from build123d import *

# Parameters (mm, degrees)
SKETCH_1_W          = 220
SKETCH_1_H          = 70
EXTRUDE_1_DEPTH     = 30
SKETCH_2_W          = 190
SKETCH_2_H          = 50
CUT_EXTRUDE_1_DEPTH = 30
SKETCH_3_W          = 20
SKETCH_3_H          = 40
CUT_EXTRUDE_2_DEPTH = 30
CUT_EXTRUDE_3_DEPTH = 30
SKETCH_5_W          = 20
SKETCH_5_H          = 60
CUT_EXTRUDE_4_DEPTH = 30
SKETCH_6_W          = 20
SKETCH_6_H          = 20
CUT_EXTRUDE_5_DEPTH = 30
SKETCH_7_W          = 20
SKETCH_7_H          = 20
CUT_EXTRUDE_6_DEPTH = 10
FILLET_1_R          = 20
EXTRUDE_2_DEPTH     = 22
EXTRUDE_3_DEPTH     = 10
EXTRUDE_START       = 10
EXTRUDE_4_DEPTH     = 10
CUT_EXTRUDE_7_DEPTH = 10
CUT_EXTRUDE_8_DEPTH = 299


with BuildPart() as part:
    # 草图1 → 凸台-拉伸1 (new body)
    with BuildSketch(Plane.XY):
        Rectangle(SKETCH_1_W, SKETCH_1_H)
    extrude(amount=EXTRUDE_1_DEPTH)

    # 草图2 → 切除-拉伸1 (cut)
    with BuildSketch(Plane.XY.offset(30)):
        with Locations((15, -10)):
            Rectangle(SKETCH_2_W, SKETCH_2_H)
    extrude(amount=-CUT_EXTRUDE_1_DEPTH, mode=Mode.SUBTRACT)

    # 草图3 → 切除-拉伸2 (cut)
    with BuildSketch(Plane(origin=(-80, 0, 0), x_dir=(0, 0, -1), z_dir=(1, 0, 0))):
        with Locations((-15, -35)):
            Rectangle(SKETCH_3_W, SKETCH_3_H)
    extrude(amount=-CUT_EXTRUDE_2_DEPTH, mode=Mode.SUBTRACT)

    # 草图4 → 切除-拉伸3 (cut)
    with BuildSketch(Plane.XY.offset(30)):
        Polygon((110, 35), (90, 15), (110, 15), align=None)
    extrude(amount=-CUT_EXTRUDE_3_DEPTH, mode=Mode.SUBTRACT)

    # 草图5 → 切除-拉伸4 (cut)
    with BuildSketch(Plane(origin=(37.5, -37.5, 0), x_dir=(0, 0, -1), z_dir=(0.7071067811865536, -0.7071067811865415, 0))):
        with Locations((-15, 102.530483272)):
            Rectangle(SKETCH_5_W, SKETCH_5_H)
    extrude(amount=-CUT_EXTRUDE_4_DEPTH, mode=Mode.SUBTRACT)

    # 草图6 → 切除-拉伸5 (cut)
    with BuildSketch(Plane(origin=(0, 35, 0), x_dir=(1, 0, 0), z_dir=(0, 1, 0))):
        with Locations((77.573593129, -15)):
            Rectangle(SKETCH_6_W, SKETCH_6_H)
    extrude(amount=-CUT_EXTRUDE_5_DEPTH, mode=Mode.SUBTRACT)

    # 草图7 → 切除-拉伸6 (cut)
    with BuildSketch(Plane(origin=(67.573593129, 0, 0), x_dir=(0, 0, -1), z_dir=(1, 0, 0))):
        with Locations((-15, 25)):
            Rectangle(SKETCH_7_W, SKETCH_7_H)
    extrude(amount=-CUT_EXTRUDE_6_DEPTH, mode=Mode.SUBTRACT)

    # 圆角1
    fillet_1_edges = [part.edges().sort_by_distance(p)[0] for p in [
        (-80, 15, 15),
    ]]
    fillet(fillet_1_edges, radius=FILLET_1_R)

    # 草图8 → 凸台-拉伸2 (add)
    with BuildSketch(Plane(origin=(0, 0, 25), x_dir=(-1, 0, 0), z_dir=(0, 0, -1))):
        Polygon((-57.573593129, 15), (-77.573593129, 35), (-57.573593129, 35), align=None)
    extrude(amount=EXTRUDE_2_DEPTH)

    # 草图9 → 凸台-拉伸3 (add)
    with BuildSketch(Plane.XY.offset(30)):
        with BuildLine():
            Line((90, 15), (110, 35))
            Line((110, 35), (-110, 35))
            Line((-110, 35), (-110, -35))
            Line((-110, -35), (-80, -35))
            Line((-80, -35), (-80, -5))
            ThreePointArc((-80, -5), (-74.142135624, 9.142135624), (-60, 15))
            Line((-60, 15), (90, 15))
        make_face()
    extrude(amount=EXTRUDE_3_DEPTH)

    # 草图10 → 凸台-拉伸4 (add)
    with BuildSketch(Plane(origin=(0, 0, 0), x_dir=(-1, 0, 0), z_dir=(0, 0, -1)).offset(EXTRUDE_START)):
        with BuildLine():
            Line((110, 35), (-110, 35))
            Line((-110, 35), (-90, 15))
            Line((-90, 15), (60, 15))
            ThreePointArc((60, 15), (74.142135624, 9.142135624), (80, -5))
            Line((80, -5), (80, -35))
            Line((80, -35), (110, -35))
            Line((110, -35), (110, 35))
        make_face()
    extrude(amount=-EXTRUDE_4_DEPTH)

    # 草图11 → 切除-拉伸7 (cut)
    with BuildSketch(Plane.XZ.offset(-15)):
        with BuildLine():
            Line((-47.5, 25), (37.5, 25))
            ThreePointArc((37.5, 25), (47.5, 15), (37.5, 5))
            Line((37.5, 5), (-47.5, 5))
            ThreePointArc((-47.5, 5), (-57.5, 15), (-47.5, 25))
        make_face()
    extrude(amount=-CUT_EXTRUDE_7_DEPTH, mode=Mode.SUBTRACT)

    # 草图12 → 切除-拉伸8 (cut)
    with BuildSketch(Plane.ZY.offset(110)):
        Polygon((-10, 31), (-5, 26), (-10, 21), align=None)
        Polygon((40, 31), (35, 26), (40, 21), align=None)
    extrude(amount=-CUT_EXTRUDE_8_DEPTH, mode=Mode.SUBTRACT)


solid = part.part
Geometry check sheet. Reference: the model listing, model coordinates, mm. A direction names the side the tool comes from. Give positions to 0.01 mm unless a question says otherwise; leave off trailing zeros. Order: outer loops, then holes, each group sorted by start corner. A loop starts at its lowest first (then second) coordinate and runs counter-clockwise, first axis right, second up.
1. Sectioned sample at A-A (y = -23). Record the boundary of the cut face in (x, z), then the cut area to 3 significant figures.
Completed:
outline: (-110, -10) - (-80, -10) - (-80, 5) - (-110, 5) - close; (-110, 25) - (-80, 25) - (-80, 40) - (-110, 40) - close
area: 900 mm2
2. Sectioned sample at B-B (z = -3). Record the boundary of the cut face in (x, y).
Completed:
outline: (-110, -35) - (-80, -35) - (-80, -5) arc R20 cw to (-60, 15) - (90, 15) - (110, 35) - (-110, 35) - close
3. Depth check by flat-ended pin: pin 1 (6 mm diameter, centred on x = -97, z = 19, fed in from -Y); pin 2 (5 mm diameter, centred on x = -6, y = 21.5, fed in from -Z); pin 3 (10 mm diameter, centred on x = 21, z = 17.5, fed in from -Y); pin 4 (8 mm diameter, centred on x = -60.5, z = 17.5, fed in from -Y). Enter the tip coordinate at first touch or a pass-through.
Completed:
pin 1: stops at y = -15
pin 2: stops at z = -10
pin 3: stops at y = 25
pin 4: stops at y = 14.49
4. Draft check along Z on faces 1 (the face through (2, 33, -10)), 2 (the face through (-95, -35, 32)), 3 (the face through (67.434, 24.86, 15.14)). Enter one of: pulls with the +Z half, pulls with the -Z half, needs draft (parallel to the pull), parting line crosses it, or undercut.
Completed:
face 1: pulls with the -Z half
face 2: needs draft
face 3: undercut
5. Sectioned sample at D-D (z = 15). Record the boundary of the cut face in (x, y), then the cut area to 3 significant figures.
Completed:
outline: (-110, -15) - (-80, -15) - (-80, -5) arc R20 cw to (-60, 15) - (-57.5, 15) - (-57.5, 25) - (47.5, 25) - (47.5, 15) - (57.57, 15) - (77.57, 35) - (-110, 35) - close
area: 3,490 mm2
6. Access from +Z, -Z, +X, -X, +Y, -Y to the whole of each face (thin tool, end or side, straight path). Record for faces 4 (the face through (-4, 20, 5)), 5 (the face through (-80, -13, 15)), 6 (the face through (84, 25, 25)), 7 (the face through (-95, -25, 25)), 8 (the face through (-4, 29, 38)).
Completed:
face 4: -Y
face 5: +Z, -Z, +X, -Y
face 6: +X, -Y
face 7: +X, -X, -Y
face 8: +Z, +X, -X
7. Scan lines: line 1 (Y direction, x = -41.5, z = 36.5); line 2 (Y direction, x = -24.5, z = 29); line 3 (Z direction, x = 81.5, y = 32). Record each from-to range of solid material in increasing order.
Completed:
line 1: y = 15 to 24.5, 27.5 to 35
line 2: y = 15 to 35
line 3: z = -10 to 5, 25 to 40
8. Sectioned sample at C-C (x = 73.5). Record the boundary of the cut face in (y, z).
Completed:
outline: (15, -10) - (21, -10) - (26, -5) - (31, -10) - (35, -10) - (35, 40) - (31, 40) - (26, 35) - (21, 40) - (15, 40) - (15, 25) - (30.93, 25) - (30.93, 5) - (15, 5) - close
